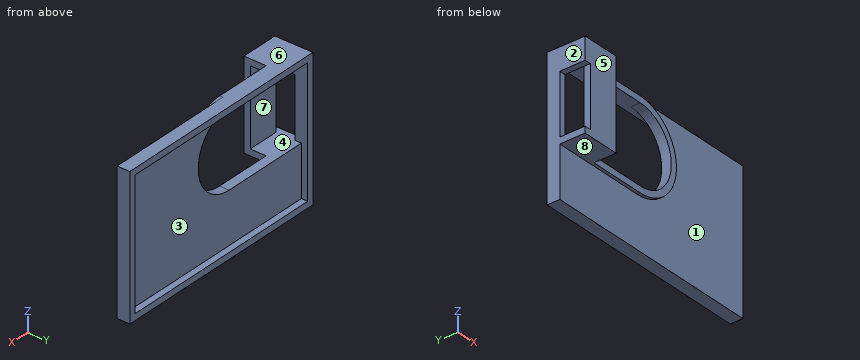
```python
from build123d import *

# Parameters (mm, degrees)
SKETCH1_W           = 67
SKETCH1_H           = 40
BOSS_EXTRUDE1_DEPTH = 2
SKETCH1_3_W         = 71
SKETCH1_3_H         = 44
SKETCH1_3_W_2       = 67
SKETCH1_3_H_2       = 40
BOSS_EXTRUDE2_DEPTH = 4
SKETCH1_5_W         = 28
SKETCH1_5_H         = 24
CUT_EXTRUDE4_DEPTH  = 2
SKETCH2_W           = 12
SKETCH2_H           = 2
BOSS_EXTRUDE3_DEPTH = 8
SKETCH3_W           = 10
SKETCH3_H           = 2
BOSS_EXTRUDE4_DEPTH = 24
BOSS_EXTRUDE5_START = 1
BOSS_EXTRUDE5_DEPTH = 1


with BuildPart() as part:
    # Sketch1 → Boss-Extrude1 (new body)
    with BuildSketch(Plane(origin=(0, 0, 0), x_dir=(1, 0, 0), z_dir=(0, 1, 0))):
        with Locations((33.5, -20)):
            Rectangle(SKETCH1_W, SKETCH1_H)
    extrude(amount=BOSS_EXTRUDE1_DEPTH)

    # Sketch1<3> → Boss-Extrude2 (add)
    with BuildSketch(Plane(origin=(0, 0, 0), x_dir=(1, 0, 0), z_dir=(0, 1, 0))):
        with Locations((33.5, -20)):
            Rectangle(SKETCH1_3_W, SKETCH1_3_H)
        with Locations((33.5, -20)):
            Rectangle(SKETCH1_3_W_2, SKETCH1_3_H_2, mode=Mode.SUBTRACT)
    extrude(amount=BOSS_EXTRUDE2_DEPTH)

    # Sketch1<5> → Cut-Extrude4 (cut)
    with BuildSketch(Plane(origin=(0, 0, 0), x_dir=(1, 0, 0), z_dir=(0, 1, 0))):
        with Locations((14, -28)):
            Rectangle(SKETCH1_5_W, SKETCH1_5_H)
        with BuildLine():
            ThreePointArc((28, -16), (40, -28), (28, -40))
            Line((28, -40), (28, -16))
        make_face()
    extrude(amount=CUT_EXTRUDE4_DEPTH, mode=Mode.SUBTRACT)

    # Sketch2 → Boss-Extrude3 (add)
    with BuildSketch(Plane.XZ):
        with Locations((4, 15)):
            Rectangle(SKETCH2_W, SKETCH2_H)
        Polygon((-2, 42), (10, 42), (10, 40), (0, 40), (0, 35), (-2, 35), (-2, 40), align=None)
    extrude(amount=BOSS_EXTRUDE3_DEPTH)

    # Sketch3 → Boss-Extrude4 (add)
    with BuildSketch(Plane(origin=(0, 0, 40), x_dir=(-1, 0, 0), z_dir=(0, 0, -1))):
        with Locations((-5, -7)):
            Rectangle(SKETCH3_W, SKETCH3_H)
    extrude(amount=BOSS_EXTRUDE4_DEPTH)

    # Sketch5 → Boss-Extrude5 (add)
    with BuildSketch(Plane.XZ.offset(BOSS_EXTRUDE5_START)):
        with BuildLine():
            Line((10, 16), (28, 16))
            ThreePointArc((28, 16), (40, 28), (28, 40))
            Line((28, 40), (10, 40))
            Line((10, 40), (10, 42))
            Line((10, 42), (28, 42))
            ThreePointArc((28, 42), (42, 28), (28, 14))
            Line((28, 14), (10, 14))
            Line((10, 14), (10, 16))
        make_face()
    extrude(amount=-BOSS_EXTRUDE5_DEPTH)


solid = part.part
```
Design review of the part built by this model. Coordinates are the model's own, in mm. Face numbers are marked on the shaded views. A direction names the side the tool comes from. Coordinates: 2 decimals unless noted, no trailing zeros. Loops run counter-clockwise (first coordinate to the right, second up) from the corner with the lowest first, then second, coordinate; pieces in that order, holes last. Notation, with made-up numbers: (32.5, 44.5) -> (63.5, 44.5) arc R27 ccw to (63.5, 75.5) -> close; hole circle Ø4 at (33.5, -1). An arc over 180 degrees is marked (long way). Answer as a JSON object with one key per item and string values.
Q1. Take a section at C-C on y = -3.25. Give the boundary of the cut face in (x, z).
Answer block:
{"outline": "(-2, 14) -> (10, 14) -> (10, 16) -> (-2, 16) -> close; (-2, 35) -> (0, 35) -> (0, 40) -> (10, 40) -> (10, 42) -> (-2, 42) -> close"}
Q2. Take a section at D-D on x = 52.5. Give the boundary of the cut face in (y, z).
Answer block:
{"outline": "(0, -2) -> (4, -2) -> (4, 0) -> (2, 0) -> (2, 40) -> (4, 40) -> (4, 42) -> (0, 42) -> close"}
Q3. Take a section at A-A on z = 28. Give the boundary of the cut face in (x, y), plus the area to 3 significant figures.
Answer block:
{"outline": "(-2, 0) -> (0, 0) -> (0, 4) -> (-2, 4) -> close; (0, -8) -> (10, -8) -> (10, -6) -> (0, -6) -> close; (40, -1) -> (42, -1) -> (42, 0) -> (69, 0) -> (69, 4) -> (67, 4) -> (67, 2) -> (40, 2) -> close", "area": "92.0 mm^2"}
Q4. Clearance check with flat-ended pins moving along their axes: pin 1 Ø1.6 at (y, z) = (-6.5, 27) entering from -X; pin 2 Ø1.6 at (x, y) = (-1, -3.5) entering from -Z; pin 3 Ø3 at (x, z) = (5, 34) entering from +Y. State where each tip first meets the part, or that it passes through.
Answer block:
{"pin 1": "stops at x = 0", "pin 2": "stops at z = 14", "pin 3": "stops at y = -6"}
Q5. The part is to be moulded in two halves that separate along X. For the marked faces 1, 2 and 3, say which applies: +X half, -X half, draft (parallel to the pull), parting line (faces both ways), or undercut.
Answer block:
{"face 1": "draft", "face 2": "-X half", "face 3": "undercut"}
Q6. To check wall thickness, follow L1, parallel to Z at x = 8.5, y = -3.25; L2, parallel to X at y = 2.5, z = 1; L3, parallel to Z at x = 28, y = 1.25. State the ranges of each line that lie inside material, in increasing order.
Answer block:
{"L1": "z = 14 to 16, 40 to 42", "L2": "x = -2 to 0, 67 to 69", "L3": "z = -2 to 16, 40 to 42"}
Q7. Tool access review of the marked faces 4, 5, 6, 7 and 8: name each direction out of +Z, -Z, +X, -X, +Y, -Y from which nothing blocks a thin tool from reaching the whole face with its end or side.
Answer block:
{"face 4": "none", "face 5": "+Z, -Z, +X, -X, -Y", "face 6": "+Z, +X, -X, +Y, -Y", "face 7": "+X, +Y", "face 8": "-Z, +X, -X, -Y"}
Q8. Take a section at B-B on x = 20. Give the boundary of the cut face in (y, z), plus the area to 3 significant figures.
Answer block:
{"outline": "(-1, 14) -> (0, 14) -> (0, -2) -> (4, -2) -> (4, 0) -> (2, 0) -> (2, 16) -> (-1, 16) -> close; (-1, 40) -> (4, 40) -> (4, 42) -> (-1, 42) -> close", "area": "52.0 mm^2"}
